Check sheet for the modelled part. Datum: model origin and axes. Units: mm. Give positions to 0.01 mm unless a question says otherwise; leave off trailing zeros. Loops run counter-clockwise (first coordinate to the right, second up) from the corner with the lowest first, then second, coordinate; pieces in that order, holes last. Notation, with made-up numbers: (-35.5, -33) - (19.5, -33) arc R22 cw to (19.5, -19) - close; hole circle Ø3 at (71, 12). An arc over 180 degrees is marked (long way). Use CSV: the item, a comma, the result in double quotes.
from build123d import *

# Parameters (mm, degrees)
F0_R     = 4.8652202412
F0_W     = 76.2
F0_H     = 12.7
F1_DEPTH = 6.35


# Not quite as in the source:
# - a length typed as a fraction of an inch, garbled in the dataset ("3 / 203.2 mm" for 3/8 in), is restored
# - a feature names something its author has since deleted; it is built from what else it names


with BuildPart() as f1:
    # F0 (on Right) → F1 (new body)
    with BuildSketch(Plane.YZ):
        Polygon((63.5, 7.14375), (-63.5, 7.14375), (-63.5, -7.14375), (12.7, -7.14375), (63.5, -7.14375), align=None)
        Polygon((63.5, -32.54375), (63.5, -7.14375), (12.7, -7.14375), (12.7, -19.84375), (12.7, -32.54375), align=None)
        with Locations((19.9129190296, -13.6523451656)):
            Circle(F0_R, mode=Mode.SUBTRACT)
        with Locations((-25.4, -13.49375)):
            Rectangle(F0_W, F0_H)
    extrude(amount=-F1_DEPTH)


solid = f1.part
1. Scan lines: line 1 along Z through (x, y) = (-0.5, -9.5); line 2 along Y through (x, z) = (-4.5, -27); line 3 along Y through (x, z) = (-0.75, -12). Record each from-to range of solid material in increasing order.
Completed:
line 1,"z = -19.84 to 7.14"
line 2,"y = 12.7 to 63.5"
line 3,"y = -63.5 to 15.34, 24.49 to 63.5"
2. Sectioned sample at D-D, the plane z = -24. Record the boundary of the cut face in (x, y).
Completed:
outline,"(-6.35, 12.7) - (0, 12.7) - (0, 63.5) - (-6.35, 63.5) - close"
3. Release check for a two-part mould opening along Z. For faces 1 (the face through (-3, 1, 7.144)), 2 (the face through (-3, 12.7, -26)), 3 (the face through (-3.131, 18.858, -18.402)), 4 (the face through (-3, -26, -19.844)) record: released by +Z, released by -Z, zero draft, split by the parting line, or undercut.
Completed:
face 1,"released by +Z"
face 2,"zero draft"
face 3,"undercut"
face 4,"released by -Z"
4. Go/stop test with a flat-tipped pin: pin 1 Ø1 at (x, z) = (-2.5, -24.5) entering from -Y. Record where the tip stops, or that it passes through.
Completed:
pin 1,"stops at y = 12.7"
5. Sectioned sample at B-B, the plane x = -3.25. Record the boundary of the cut face in (y, z), and give its area (3 significant figures).
Completed:
outline,"(-63.5, -19.84) - (12.7, -19.84) - (12.7, -32.54) - (63.5, -32.54) - (63.5, 7.14) - (-63.5, 7.14) - close; hole circle Ø9.73 at (19.91, -13.65)"
area,"4,000 mm²"
6. Sectioned sample at A-A, the plane z = -15. Record the boundary of the cut face in (x, y), and give its area (3 significant figures).
Completed:
outline,"(-6.35, -63.5) - (0, -63.5) - (0, 15.24) - (-6.35, 15.24) - close; (-6.35, 24.59) - (0, 24.59) - (0, 63.5) - (-6.35, 63.5) - close"
area,"747 mm²"
7. Sectioned sample at C-C, the plane y = -4. Record the boundary of the cut face in (x, z).
Completed:
outline,"(-6.35, -19.84) - (0, -19.84) - (0, 7.14) - (-6.35, 7.14) - close"
